Geometry check sheet. Reference: the model listing, model coordinates, mm. Face numbers are marked on the shaded views. Coordinates: 2 decimals unless noted, no trailing zeros. Write each loop counter-clockwise with the first axis right and the second up, starting at its lowest first coordinate (ties: lowest second). Pieces come first, ordered by that corner, then holes. Notation, with made-up numbers: (14, 62.25) -> (69, 62.25) arc R29 cw to (69, 83.25) -> close; hole circle Ø11 at (-30, -29.5). An arc over 180 degrees is marked (long way). Use a Markdown table: item, result.
```python
from build123d import *

# Parameters (mm, degrees)
SKETCH1_R                                    = 2
SKETCH1_R_2                                  = 6
BOSS_EXTRUDE1_DEPTH                          = 3
FILLET1_R                                    = 5
CSK_FOR_M4_COUNTERSUNK_FLAT_HEAD_SCR_2_COUNT = 2
CSK_FOR_M4_COUNTERSUNK_FLAT_HEAD_SCR_2_PITCH = 23.508708273
CSK_FOR_M5_COUNTERSUNK_FLAT_HEAD_SCR_2_COUNT = 2
CSK_FOR_M5_COUNTERSUNK_FLAT_HEAD_SCR_2_PITCH = 50.8


with BuildPart() as part:
    # Sketch1 → Boss-Extrude1 (new body)
    with BuildSketch(Plane.XY):
        with BuildLine():
            Line((16.48489132, -19.999559574), (2.484638151, -8.650235445))
            ThreePointArc((2.484638151, -8.650235445), (-5.667544957, -6.991347092), (-8.977125763, 0.641258943))
            Line((-8.977125763, 0.641258943), (-22.977378932, 11.990583072))
            ThreePointArc((-22.977378932, 11.990583072), (-24.590001349, 17.71711779), (-19.731135126, 21.150071323))
            Line((-19.731135126, 21.150071323), (-14.065364661, 21.150071323))
            Line((-14.065364661, 21.150071323), (-13.75, 21.150071323))
            Line((-13.75, 21.150071323), (-13.75, 34.45))
            Line((-13.75, 34.45), (13.75, 34.45))
            Line((13.75, 34.45), (36.75, 34.45))
            ThreePointArc((36.75, 34.45), (45.726790692, 24.804067443), (35.461466363, 16.542717526))
            ThreePointArc((35.461466363, 16.542717526), (18.351015207, 7.031288175), (22.977378932, -11.990583072))
            ThreePointArc((22.977378932, -11.990583072), (23.735623377, -19.241315129), (16.48489132, -19.999559574))
        make_face()
        with Locations((-19.731135126, 15.995071323)):
            Circle(SKETCH1_R, mode=Mode.SUBTRACT)
        with Locations((19.731135126, -15.995071323)):
            Circle(SKETCH1_R, mode=Mode.SUBTRACT)
        Circle(SKETCH1_R_2, mode=Mode.SUBTRACT)
        with Locations((36.75, 25.45)):
            Circle(SKETCH1_R_2, mode=Mode.SUBTRACT)
    extrude(amount=BOSS_EXTRUDE1_DEPTH)

    # Fillet1
    fillet1_edges = [part.edges().sort_by_distance(p)[0] for p in [
        (2.484638151, -8.650235445, 1.5),
        (-8.977125763, 0.641258943, 1.5),
        (-13.75, 21.150071323, 1.5),
        (-13.75, 34.45, 1.5),
    ]]
    fillet(fillet1_edges, radius=FILLET1_R)

    # Sketch3 → CSK for M4 Countersunk Flat Head Screw1 (revolve, cut)
    with BuildSketch(Plane(origin=(13.75, 29.45, 0), x_dir=(0, 1, 0), z_dir=(1, 0, 0))):
        Polygon((0, 0), (0, 3), (2.25, 3), (2.25, 2.45), (4.7, 0), align=None)
    csk_for_m4_countersunk_flat_head_screw1 = revolve(axis=Axis((13.75, 29.45, -6.35), (0, 0, 1)), mode=Mode.SUBTRACT)

    # CSK for M4 Countersunk Flat Head Scr 2: CSK for M4 Countersunk Flat Head Screw1 ×2
    with Locations(*[(-i * CSK_FOR_M4_COUNTERSUNK_FLAT_HEAD_SCR_2_PITCH, 0, 0) for i in range(1, CSK_FOR_M4_COUNTERSUNK_FLAT_HEAD_SCR_2_COUNT)]):
        add(csk_for_m4_countersunk_flat_head_screw1, mode=Mode.SUBTRACT)

    # Sketch6 → CSK for M5 Countersunk Flat Head Screw1 (revolve, cut)
    with BuildSketch(Plane(origin=(-19.731135126, 15.995071323, 3), x_dir=(0, -1, 0), z_dir=(1, 0, 0))):
        Polygon((0, 0), (0, 3), (2.75, 3), (2.75, 2.45), (5.2, 0), align=None)
    csk_for_m5_countersunk_flat_head_screw1 = revolve(axis=Axis((-19.731135126, 15.995071323, 9.35), (0, 0, -1)), mode=Mode.SUBTRACT)

    # CSK for M5 Countersunk Flat Head Scr 2: CSK for M5 Countersunk Flat Head Screw1 ×2
    with Locations(*[Vector(0.7768163435563247, -0.6297272174392513, 0) * (i * CSK_FOR_M5_COUNTERSUNK_FLAT_HEAD_SCR_2_PITCH) for i in range(1, CSK_FOR_M5_COUNTERSUNK_FLAT_HEAD_SCR_2_COUNT)]):
        add(csk_for_m5_countersunk_flat_head_screw1, mode=Mode.SUBTRACT)


solid = part.part
```
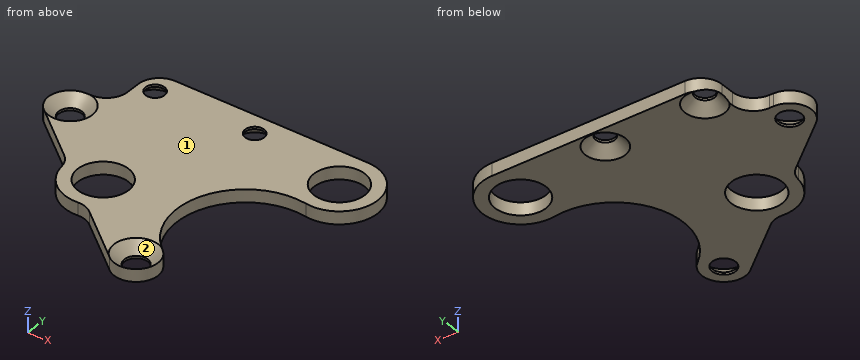
Item 1: Section check B-B on z = 1.5. Record the boundary of the cut face in (x, y) (3 decimals), then the cut area to 3 significant figures.
Answer block:
| item | result |
|---|---|
| outline | (-22.977, 11.991) -> (-10.733, 2.064) arc R5 cw to (-8.924, -1.17) arc R9 ccw to (0.702, -8.973) arc R5 cw to (4.24, -10.073) -> (16.485, -20) arc R5.155 ccw to (22.977, -11.991) arc R16.152 cw to (35.461, 16.543) arc R9 ccw (long way) to (36.75, 34.45) -> (-8.75, 34.45) arc R5 ccw to (-13.75, 29.45) -> (-13.75, 26.15) arc R5 cw to (-18.75, 21.15) -> (-19.731, 21.15) arc R5.155 ccw to start; hole circle Ø7.4 at (-19.731, 15.995); hole circle Ø6.4 at (-9.759, 29.45); hole circle Ø12 at (0, 0); hole circle Ø6.4 at (13.75, 29.45); hole circle Ø7.4 at (19.731, -15.995); hole circle Ø12 at (36.75, 25.45) |
| area | 1,720 mm^2 |
Item 2: Section check C-C on x = -3.5. Record the boundary of the cut face in (y, z).
Answer block:
| item | result |
|---|---|
| outline | (-8.29, 0) -> (-4.87, 0) -> (-4.87, 3) -> (-8.29, 3) -> close; (4.87, 0) -> (34.45, 0) -> (34.45, 3) -> (4.87, 3) -> close |
Item 3: Mould release check, pull along Y, two halves, no side actions. Record for the marked faces 1 and 2: +Y half, -Y half, draft (parallel to the pull), parting line (faces both ways), or undercut.
Answer block:
| item | result |
|---|---|
| face 1 | draft |
| face 2 | undercut |
Item 4: Depth check by flat-ended pin: P1, Ø0.9, axis at y = 28, z = 1.5, coming from the -X side; P2, Ø1.5, axis at x = 3.5, z = 2, coming from the -Y side; P3, Ø6.5, axis at x = 19.73, y = -16, coming from the +Z side; P4, Ø3.5, axis at x = -9.76, y = 29.45, coming from the -Z side. Enter the tip coordinate at first touch or a pass-through.
Answer block:
| item | result |
|---|---|
| P1 | stops at x = -13.75 |
| P2 | stops at y = -10.08 |
| P3 | stops at z = 1.06 |
| P4 | passes through |
Item 5: Section check A-A on x = 41. Record the boundary of the cut face in (y, z).
Answer block:
| item | result |
|---|---|
| outline | (17.52, 0) -> (21.21, 0) -> (21.21, 3) -> (17.52, 3) -> close; (29.69, 0) -> (33.38, 0) -> (33.38, 3) -> (29.69, 3) -> close |
Item 6: Thickness scan on L1, parallel to Y at x = 36.75, z = 0.9; L2, parallel to Y at x = 0, z = 2; L3, parallel to X at y = -13.5, z = 2.45. Record the ranges inside material, lowest first. Write a range as [from, to].
Answer block:
| item | result |
|---|---|
| L1 | y = [16.45, 19.45], [31.45, 34.45] |
| L2 | y = [-9, -6], [6, 34.45] |
| L3 | x = [8.47, 15.81], [23.66, 24.24] |
Item 7: Section check D-D on y = -8. Record the boundary of the cut face in (x, z), then the cut area to 3 significant figures.
Answer block:
| item | result |
|---|---|
| outline | (-4.12, 0) -> (19.45, 0) -> (19.45, 3) -> (-4.12, 3) -> close |
| area | 70.7 mm^2 |
